The listing builds one solid part. Answer for the finished solid, in the listing's coordinates (mm). A direction names the side the tool comes from. Coordinates: 2 decimals unless noted, no trailing zeros. Order: outer loops, then holes, each group sorted by start corner. A loop starts at its lowest first (then second) coordinate and runs counter-clockwise, first axis right, second up. Notation, with made-up numbers: (50, 83.5) -> (58, 83.5) arc R16 ccw to (58, 109.5) -> close; hole circle Ø9 at (45.25, 66). An arc over 180 degrees is marked (long way). Answer in a Markdown table with one row per item. Add a question column.
```python
from build123d import *

# Parameters (mm, degrees)
BOSS_EXTRUDE1_DEPTH = 15
CUT_EXTRUDE1_DEPTH  = 37.5


with BuildPart() as part:
    # Sketch1 → Boss-Extrude1 (new body)
    with BuildSketch(Plane(origin=(0, 0, 0), x_dir=(1, 0, 0), z_dir=(0, 1, 0))):
        Polygon((32.5, -60), (37.5, -60), (37.5, 60), (-37.5, 60), (-37.5, -60), (-32.5, -60), (-32.5, 40), (32.5, 40), align=None)
    extrude(amount=BOSS_EXTRUDE1_DEPTH)

    # Sketch2 → Cut-Extrude1 (cut, symmetric)
    with BuildSketch(Plane(origin=(0, 0, 0), x_dir=(0, 0, -1), z_dir=(1, 0, 0))):
        Polygon((-60, 11), (-25, 11), (-20, 8.877625919), (-20, 7.575525184), (-24, 7.575525184), (-25, 8), (-60, 8), align=None)
    extrude(amount=CUT_EXTRUDE1_DEPTH, both=True, mode=Mode.SUBTRACT)


solid = part.part
```
Q1. A cutting plane is placed at C-C (y = 13). Determine the outline of the cut face in (x, z), then the cut area to 3 significant figures.
Q2. A cutting plane is placed at B-B (z = 32). Determine the outline of the cut face in (x, y).
Q3. Determine the mould class of faces 6 (the face through (-1, 15, -41)), 7 (the face through (-1, 0, -41)), 8 (the face through (-35, 11, 43)) for opening direction Y: +Y half, -Y half, draft (parallel to the pull), parting line (faces both ways), or undercut.
Q4. For faces 1 (the face through (1, 7, -60)), 2 (the face through (-35, 7.576, 22)), 3 (the face through (-35, 8, 42)), 4 (the face through (35, 4, 60)), 5 (the face through (0, 7, -40)), determine the directions among +Z, -Z, +X, -X, +Y, -Y from which every point of the face is accessible in a straight line to the end or side of a thin tool.
Q5. A cutting plane is placed at D-D (x = -4.5). Determine the outline of the cut face in (y, z).
Q6. A cutting plane is placed at A-A (z = -26). Determine the outline of the cut face in (x, y).
Q7. Straight lines are drawn through the part: line 1 (X direction, y = 6.75, z = 4.5); line 2 (Z direction, x = 9.5, y = 6.75). For each, find the intervals that lie inside material, in ascending order.
Q8. Given pin 1 (1.5 mm diameter, centred on x = -27.5, y = 8, fed in from +Z); pin 2 (0.7 mm diameter, centred on x = -35, y = 8.5, fed in from +Z), each flat-ended and moving along its own axis, determine where each tip first touches the part or whether it passes through.
Returned:
| question | item | result |
|---|---|---|
| 1 | outline | (-37.5, -60) -> (37.5, -60) -> (37.5, 60) -> (32.5, 60) -> (32.5, -40) -> (-32.5, -40) -> (-32.5, 60) -> (-37.5, 60) -> close |
| 1 | area | 2,500 mm² |
| 2 | outline | (-37.5, 0) -> (-32.5, 0) -> (-32.5, 8) -> (-37.5, 8) -> close; (-37.5, 11) -> (-32.5, 11) -> (-32.5, 15) -> (-37.5, 15) -> close; (32.5, 0) -> (37.5, 0) -> (37.5, 8) -> (32.5, 8) -> close; (32.5, 11) -> (37.5, 11) -> (37.5, 15) -> (32.5, 15) -> close |
| 3 | face 6 | +Y half |
| 3 | face 7 | -Y half |
| 3 | face 8 | undercut |
| 4 | face 1 | -Z, +X, -X, +Y, -Y |
| 4 | face 2 | +X, -X |
| 4 | face 3 | +Z, +X, -X |
| 4 | face 4 | +Z, +X, -X, +Y, -Y |
| 4 | face 5 | +Z, +Y, -Y |
| 5 | outline | (0, -60) -> (15, -60) -> (15, -40) -> (0, -40) -> close |
| 6 | outline | (-37.5, 0) -> (-32.5, 0) -> (-32.5, 15) -> (-37.5, 15) -> close; (32.5, 0) -> (37.5, 0) -> (37.5, 15) -> (32.5, 15) -> close |
| 7 | line 1 | x = -37.5 to -32.5, 32.5 to 37.5 |
| 7 | line 2 | z = -60 to -40 |
| 8 | pin 1 | stops at z = -40 |
| 8 | pin 2 | stops at z = 20 |
